Geometry check sheet. Reference: the model listing, model coordinates, mm. Face numbers are marked on the shaded views. Coordinates: 2 decimals unless noted, no trailing zeros. Loops run counter-clockwise (first coordinate to the right, second up) from the corner with the lowest first, then second, coordinate; pieces in that order, holes last.
from build123d import *
from build123d import SkipClean  # not in build123d's __all__

# Parameters (mm, degrees)
F0_W        = 2
F0_H        = 2
F0_H_2      = 3
F2_SIZE     = 1
F4_DEPTH    = 5
F5_DEPTH    = 3
F6_T4_DEPTH = 10.6380386618
F6_T6_DEPTH = 6.8190193309
F6_T8_DEPTH = 6.8190193309


# Not quite as in the source:
# - a fillet or chamfer that OpenCascade refuses, or shapes differently, is made with other operations: its cross-section is extruded or revolved along the edge and cut away or added


with BuildPart() as f1:
    # F0 (on Front) → F1 (revolve)
    with BuildSketch(Plane.XZ):
        Polygon((33.2, -3.5), (33.2, 3.5), (29.5090141887, 3.5), (29.5090141887, 1.5), (31.2, 1.5), (31.2, -3.5), align=None)
        with Locations((28.5090141887, 2.5)):
            Rectangle(F0_W, F0_H)
        with Locations((28.5090141887, 5)):
            Rectangle(F0_W, F0_H_2)
        Polygon((27.5090141887, 6.5), (29.5090141887, 6.5), (35, 6.5), (35, 8), (27.5090141887, 8), align=None)
    revolve(axis=Axis((0, 0, 0.081283506), (0, 0, -1)))

    # F2
    f2_edges = [f1.edges().sort_by_distance(p)[0] for p in [
        (-33.2, 0, 3.5),
        (-27.509014, 0, 1.5),
        (-29.509014, 0, 3.5),
        (-27.509014, 0, 8),
    ]]
    chamfer(f2_edges, length=F2_SIZE)

    # F3 (on face) → F4 (cut, through all)
    with BuildSketch(Plane(origin=(0, 0, -3.5), x_dir=(1, 0, 0), z_dir=(0, 0, -1))):
        with BuildLine():
            ThreePointArc((-4, -31.9505868491), (0, -32.2), (4, -31.9505868491))
            Line((4, -31.9505868491), (4, -30.9425273693))
            ThreePointArc((4, -30.9425273693), (0, -31.2), (-4, -30.9425273693))
            Line((-4, -30.9425273693), (-4, -31.9505868491))
        make_face()
        with BuildLine():
            ThreePointArc((-12.8274571452, -29.5346634176), (-8.5, -31.0578492494), (-4, -31.9505868491))
            Line((-4, -31.9505868491), (-4, -30.9425273693))
            ThreePointArc((-4, -30.9425273693), (-8.2963998779, -30.0767310236), (-12.4290889109, -28.6174378456))
            Line((-12.4290889109, -28.6174378456), (-12.8274571452, -29.5346634176))
        make_face()
        with BuildLine():
            ThreePointArc((-25.6700198771, 19.4393950397), (-27.8860180019, 16.1), (-29.6700198771, 12.5111918094))
            Line((-29.6700198771, 12.5111918094), (-28.7970147591, 12.0071620695))
            ThreePointArc((-28.7970147591, 12.0071620695), (-27.0199925981, 15.6), (-24.7970147591, 18.9353652998))
            Line((-24.7970147591, 18.9353652998), (-25.6700198771, 19.4393950397))
        make_face()
        with BuildLine():
            Line((-18.5688837101, 25.0726256655), (-19.1640402392, 25.8762354625))
            ThreePointArc((-19.1640402392, 25.8762354625), (-22.6468864369, 22.8901405569), (-25.6700198771, 19.4393950397))
            Line((-25.6700198771, 19.4393950397), (-24.7970147591, 18.9353652998))
            ThreePointArc((-24.7970147591, 18.9353652998), (-21.8990131903, 22.223258566), (-18.5688837101, 25.0726256655))
        make_face()
        with BuildLine():
            Line((30.9979726209, 3.5448121801), (31.9914973844, 3.6584279551))
            ThreePointArc((31.9914973844, 3.6584279551), (31.1468864369, 8.1677086925), (29.6700198771, 12.5111918094))
            Line((29.6700198771, 12.5111918094), (28.7970147591, 12.0071620695))
            ThreePointArc((28.7970147591, 12.0071620695), (30.1954130682, 7.8534724576), (30.9979726209, 3.5448121801))
        make_face()
        with BuildLine():
            Line((28.7970147591, 12.0071620695), (29.6700198771, 12.5111918094))
            ThreePointArc((29.6700198771, 12.5111918094), (27.8860180019, 16.1), (25.6700198771, 19.4393950397))
            Line((25.6700198771, 19.4393950397), (24.7970147591, 18.9353652998))
            ThreePointArc((24.7970147591, 18.9353652998), (27.0199925981, 15.6), (28.7970147591, 12.0071620695))
        make_face()
    extrude(amount=-F4_DEPTH, mode=Mode.SUBTRACT)

    # F3 (on face) → F5 (join)
    with BuildSketch(Plane(origin=(0, 0, -3.5), x_dir=(1, 0, 0), z_dir=(0, 0, -1))):
        with BuildLine():
            ThreePointArc((4, -31.9505868491), (24.1416652284, -21.3077450707), (32.2, 0))
            ThreePointArc((32.2, 0), (32.1478320869, 1.8321823356), (31.9914973844, 3.6584279551))
            Line((31.9914973844, 3.6584279551), (30.9979726209, 3.5448121801))
            ThreePointArc((30.9979726209, 3.5448121801), (31.1494522084, 1.775282263), (31.2, 0))
            ThreePointArc((31.2, 0), (23.4333096254, -20.5990291033), (4, -30.9425273693))
            Line((4, -30.9425273693), (4, -31.9505868491))
        make_face()
        with BuildLine():
            Line((30.9979726209, 3.5448121801), (31.9914973844, 3.6584279551))
            ThreePointArc((31.9914973844, 3.6584279551), (31.1468864369, 8.1677086925), (29.6700198771, 12.5111918094))
            Line((29.6700198771, 12.5111918094), (28.7970147591, 12.0071620695))
            ThreePointArc((28.7970147591, 12.0071620695), (30.1954130682, 7.8534724576), (30.9979726209, 3.5448121801))
        make_face()
        with BuildLine():
            ThreePointArc((-12.8274571452, -29.5346634176), (-8.5, -31.0578492494), (-4, -31.9505868491))
            Line((-4, -31.9505868491), (-4, -30.9425273693))
            ThreePointArc((-4, -30.9425273693), (-8.2963998779, -30.0767310236), (-12.4290889109, -28.6174378456))
            Line((-12.4290889109, -28.6174378456), (-12.8274571452, -29.5346634176))
        make_face()
        with BuildLine():
            Line((-18.5688837101, 25.0726256655), (-19.1640402392, 25.8762354625))
            ThreePointArc((-19.1640402392, 25.8762354625), (-22.6468864369, 22.8901405569), (-25.6700198771, 19.4393950397))
            Line((-25.6700198771, 19.4393950397), (-24.7970147591, 18.9353652998))
            ThreePointArc((-24.7970147591, 18.9353652998), (-21.8990131903, 22.223258566), (-18.5688837101, 25.0726256655))
        make_face()
    with SkipClean():  # cleaning this boolean's faces spoils the solid; the shape is the same uncleaned
        extrude(amount=-F5_DEPTH)

    # F6: fillet of radius 2 on 3 edges, made by hand


with BuildPart() as f6_tool2:
    # F6_s3 → F6_t4 (new body)
    with BuildSketch(Plane.XY.offset(-7.3190193309)):
        with BuildLine():
            ThreePointArc((-4, 31.9505868491), (-4.5929852552, 31.1331579467), (-5.5097528505, 30.7096503322))
            ThreePointArc((-5.5097528505, 30.7096503322), (-4.7563018983, 30.8353302601), (-4, 30.9425273693))
            Line((-4, 30.9425273693), (-4, 31.9505868491))
        make_face()
    extrude(amount=F6_T4_DEPTH)

    split(bisect_by=Plane.XY.offset(1.5), keep=Keep.BOTTOM)


with BuildPart() as f1_1:
    add(f1.part, clean=False)

    # F6_t1: cut F6_tool2
    add(f6_tool2.part, mode=Mode.SUBTRACT)

    # F6_s7 → F6_t6 (cut)
    with BuildSketch(Plane.XY.offset(-7.3190193309)):
        with BuildLine():
            ThreePointArc((-25.6700198771, -19.4393950397), (-24.6656130543, -19.5442208835), (-23.8404609038, -20.1264111032))
            ThreePointArc((-23.8404609038, -20.1264111032), (-24.3260283902, -19.5367434021), (-24.7970147591, -18.9353652998))
            Line((-24.7970147591, -18.9353652998), (-25.6700198771, -19.4393950397))
        make_face()
    extrude(amount=F6_T6_DEPTH, mode=Mode.SUBTRACT)

    # F6_s9 → F6_t8 (cut)
    with BuildSketch(Plane.XY.offset(-7.3190193309)):
        with BuildLine():
            ThreePointArc((29.6700198771, -12.5111918094), (29.2585983094, -11.5889370631), (29.3502137543, -10.583239229))
            ThreePointArc((29.3502137543, -10.583239229), (29.0823302885, -11.2985868581), (28.7970147591, -12.0071620695))
            Line((28.7970147591, -12.0071620695), (29.6700198771, -12.5111918094))
        make_face()
    extrude(amount=F6_T8_DEPTH, mode=Mode.SUBTRACT)


solid = f1_1.part
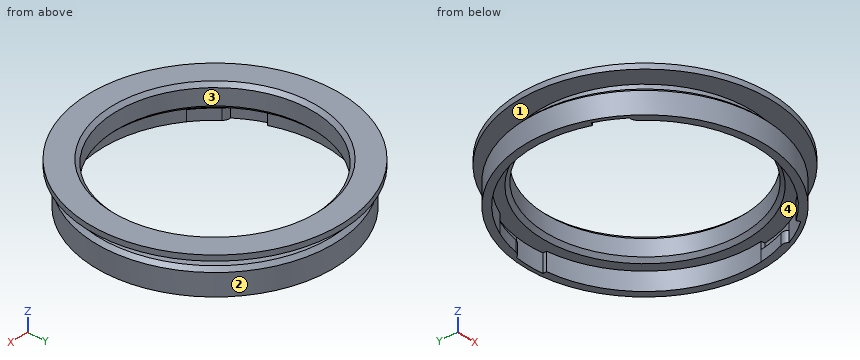
(1) Draft check along Y on the marked faces 1, 2, 3 and 4. Enter one of: +Y half, -Y half, draft (parallel to the pull), parting line (faces both ways), or undercut.
Findings:
face 1: draft
face 2: parting line
face 3: undercut
face 4: undercut
(2) Gauge pin test, flat ends, axial feed: pin 1 Ø1 at (x, z) = (23, -1.5) entering from +Y; pin 2 Ø1 at (y, z) = (20.5, -2) entering from -X; pin 3 Ø10 at (x, y) = (-23.5, -26.5) entering from -Z; pin 4 Ø5 at (y, z) = (-11, 1.5) entering from -X. Record the tip position at first contact, or that the pin passes through.
Findings:
pin 1: stops at y = 24.41
pin 2: stops at x = -26.5
pin 3: stops at z = -3.5
pin 4: stops at x = -32.09
(3) Scan lines: L1, parallel to Y at x = 0, z = 4.8; L2, parallel to Z at x = -20, y = 25. Record each from-to range of solid material in increasing order.
Findings:
L1: y = -29.51 to -27.51, 27.51 to 29.51
L2: z = -3.5 to 3.5, 6.5 to 8
(4) Sectioned sample at A-A on x = 0. Record the cut outline in (y, z).
Findings:
outline: (-35, 6.5) - (-29.51, 6.5) - (-29.51, 4.5) - (-30.51, 3.5) - (-32.2, 3.5) - (-33.2, 2.5) - (-33.2, -3.5) - (-31.2, -3.5) - (-31.2, 1.5) - (-28.51, 1.5) - (-27.51, 2.5) - (-27.51, 7) - (-28.51, 8) - (-35, 8) - close; (27.51, 2.5) - (28.51, 1.5) - (32.2, 1.5) - (32.2, -3.5) - (33.2, -3.5) - (33.2, 2.5) - (32.2, 3.5) - (30.51, 3.5) - (29.51, 4.5) - (29.51, 6.5) - (35, 6.5) - (35, 8) - (28.51, 8) - (27.51, 7) - close
(5) Sectioned sample at B-B on z = -2.5. Record the cut outline in (x, y), and give its area (3 significant figures).
Findings:
outline: circle Ø66.4 at (0, 0); hole (-29.67, -12.51) arc R32.2 ccw to (-25.67, -19.44) arc R2 cw to (-23.84, -20.13) arc R31.2 ccw to (24.8, -18.94) - (25.67, -19.44) arc R32.2 ccw to (29.67, -12.51) arc R2 cw to (29.35, -10.58) arc R31.2 ccw to (4, 30.94) - (4, 31.95) arc R32.2 ccw to (-4, 31.95) arc R2 cw to (-5.51, 30.71) arc R31.2 ccw to (-28.8, -12.01) - close
area: 379 mm2
(6) Sectioned sample at C-C on y = 0. Record the cut outline in (x, z).
Findings:
outline: (-35, 6.5) - (-29.51, 6.5) - (-29.51, 4.5) - (-30.51, 3.5) - (-32.2, 3.5) - (-33.2, 2.5) - (-33.2, -3.5) - (-31.2, -3.5) - (-31.2, 1.5) - (-28.51, 1.5) - (-27.51, 2.5) - (-27.51, 7) - (-28.51, 8) - (-35, 8) - close; (27.51, 2.5) - (28.51, 1.5) - (31.2, 1.5) - (31.2, -3.5) - (33.2, -3.5) - (33.2, 2.5) - (32.2, 3.5) - (30.51, 3.5) - (29.51, 4.5) - (29.51, 6.5) - (35, 6.5) - (35, 8) - (28.51, 8) - (27.51, 7) - close
